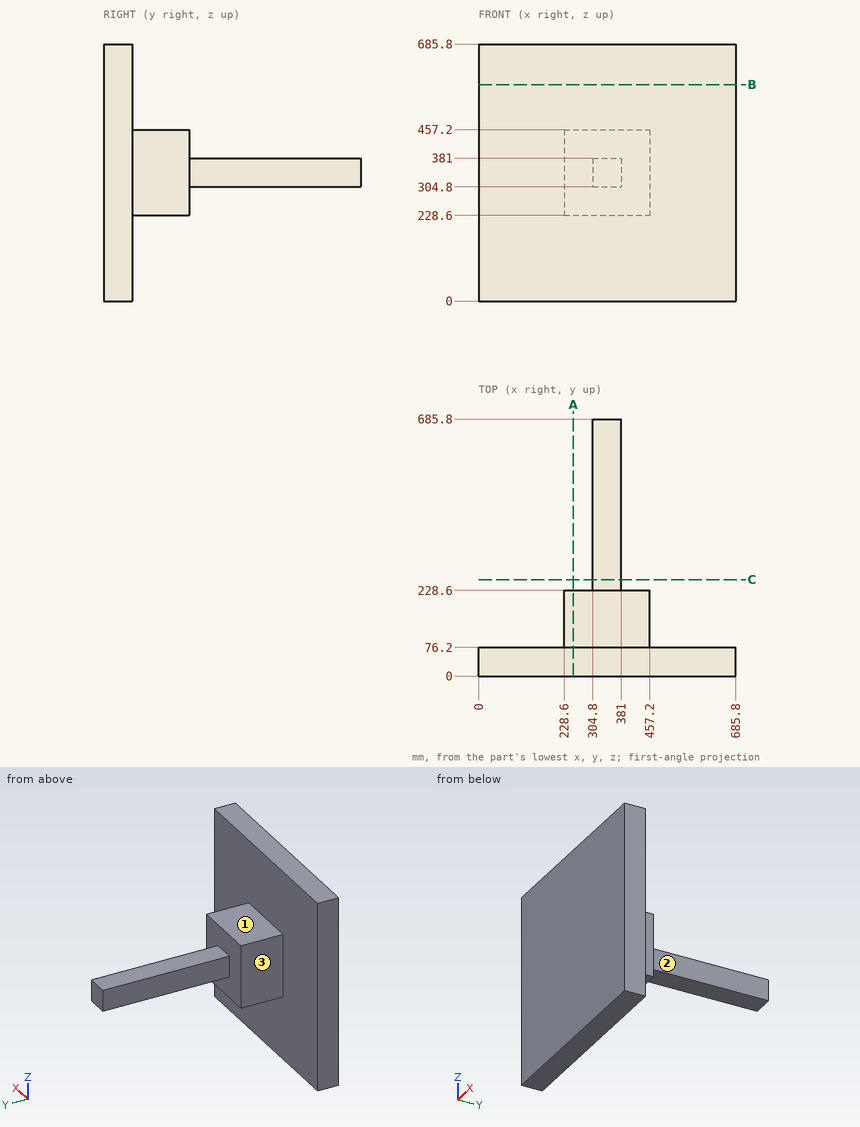
Verification items for this drawing (mm, ordinates from the low corner). A direction names the side the tool comes from. Give positions to 0.01 mm unless a question says otherwise; leave off trailing zeros. Loops run counter-clockwise (first coordinate to the right, second up) from the corner with the lowest first, then second, coordinate; pieces in that order, holes last. Notation, with made-up numbers: M 48.5,40 L 57.5,40 A6 cw 57.5,45 Z; hole C 77.5,-23.75 d2. An arc over 180 degrees is marked long. Write item = value, one per line.
(1) Sectioned sample at B-B, the plane z = 577.5. Record the cut outline in (x, y).
Answer below:
outline = M 0,0 L 685.8,0 L 685.8,76.2 L 0,76.2 Z
(2) Sectioned sample at C-C, the plane y = 257. Record the cut outline in (x, z), plus the area to 3 significant figures.
Answer below:
outline = M 304.8,304.8 L 381,304.8 L 381,381 L 304.8,381 Z
area = 5,810 mm2
(3) Sectioned sample at A-A, the plane x = 253.5. Record the cut outline in (y, z).
Answer below:
outline = M 0,0 L 76.2,0 L 76.2,228.6 L 228.6,228.6 L 228.6,457.2 L 76.2,457.2 L 76.2,685.8 L 0,685.8 Z
(4) Gauge pin test, flat ends, axial feed: pin 1 Ø5 at (y, z) = (542.5, 333) entering from -X; pin 2 Ø23 at (x, y) = (325, 477) entering from +Z; pin 3 Ø2 at (x, y) = (356.5, 473.5) entering from -Z. Record the tip position at first contact, or that the pin passes through.
Answer below:
pin_1 = 304.8
pin_2 = 381
pin_3 = 304.8
(5) Material ranges on line 1 (Y direction, x = 129, z = 57); line 2 (Z direction, x = 307.5, y = 408), recorded low to high. Write a range as [from, to].
Answer below:
line_1 = [0, 76.2]
line_2 = [304.8, 381]
(6) Tool access check on the marked faces 1, 2 and 3. Record the directions out of +Z, -Z, +X, -X, +Y, -Y that give a thin tool (end or side, any length) a straight path to the whole face; none if there is none.
Answer below:
face_1 = +Z, +X, -X, +Y
face_2 = +Z, -Z, +X, +Y
face_3 = +Z, -Z, -X, +Y
